For this review, take the finished solid that the model builds, in its own axes (mm). Face numbers are marked on the shaded views. A direction names the side the tool comes from. Coordinates: 2 decimals unless noted, no trailing zeros. Write each loop counter-clockwise with the first axis right and the second up, starting at its lowest first coordinate (ties: lowest second). Pieces come first, ordered by that corner, then holes. Notation, with made-up numbers: M 61.25,74 L 83.25,74 A31 cw 83.25,102 Z; hole C 15,-40 d8. An arc over 180 degrees is marked long. Return JSON: item names as keys, results as strings.
```python
from build123d import *

# Parameters (mm, degrees)
F0_W     = 99.4
F0_H     = 20
F1_DEPTH = 6
F2_W     = 5
F2_H     = 3.1
F2_W_2   = 6
F3_DEPTH = 6
F4_R     = 1.975
F5_DEPTH = 6
F6_W     = 30
F6_H     = 3
F7_DEPTH = 6


with BuildPart() as f1:
    # F0 (on Top) → F1 (new body)
    with BuildSketch(Plane.XY):
        Rectangle(F0_W, F0_H)
    extrude(amount=F1_DEPTH)

    # F2 (on face) → F3 (cut, through all)
    with BuildSketch(Plane.XY.offset(6)):
        with Locations((-47.2, 0)):
            Rectangle(F2_W, F2_H)
        with Locations((-41.7, 0)):
            Rectangle(F2_W_2, F2_H)
        with BuildLine():
            Line((-38.7, -1.55), (-44.7, -1.55))
            Line((-44.7, -1.55), (-44.7, -2.65))
            ThreePointArc((-44.7, -2.65), (-41.7, -5.65), (-38.7, -2.65))
            Line((-38.7, -2.65), (-38.7, -1.55))
        make_face()
        with BuildLine():
            Line((-44.7, 2.65), (-44.7, 1.55))
            Line((-44.7, 1.55), (-38.7, 1.55))
            Line((-38.7, 1.55), (-38.7, 2.65))
            ThreePointArc((-38.7, 2.65), (-41.7, 5.65), (-44.7, 2.65))
        make_face()
        with Locations((41.7, 0)):
            Rectangle(F2_W_2, F2_H)
        with BuildLine():
            Line((38.7, 2.65), (38.7, 1.55))
            Line((38.7, 1.55), (44.7, 1.55))
            Line((44.7, 1.55), (44.7, 2.65))
            ThreePointArc((44.7, 2.65), (41.7, 5.65), (38.7, 2.65))
        make_face()
        with BuildLine():
            Line((44.7, -1.55), (38.7, -1.55))
            Line((38.7, -1.55), (38.7, -2.65))
            ThreePointArc((38.7, -2.65), (41.7, -5.65), (44.7, -2.65))
            Line((44.7, -2.65), (44.7, -1.55))
        make_face()
        with Locations((47.2, 0)):
            Rectangle(F2_W, F2_H)
    extrude(amount=-F3_DEPTH, mode=Mode.SUBTRACT)

    # F4 (on face) → F5 (cut, through all)
    with BuildSketch(Plane.XY.offset(6)):
        Circle(F4_R)
    extrude(amount=-F5_DEPTH, mode=Mode.SUBTRACT)

    # F6 (on face) → F7 (cut, through all)
    with BuildSketch(Plane.XY.offset(6)):
        with Locations((-34.7, 8.5)):
            Rectangle(F6_W, F6_H)
    extrude(amount=-F7_DEPTH, mode=Mode.SUBTRACT)


solid = f1.part
```
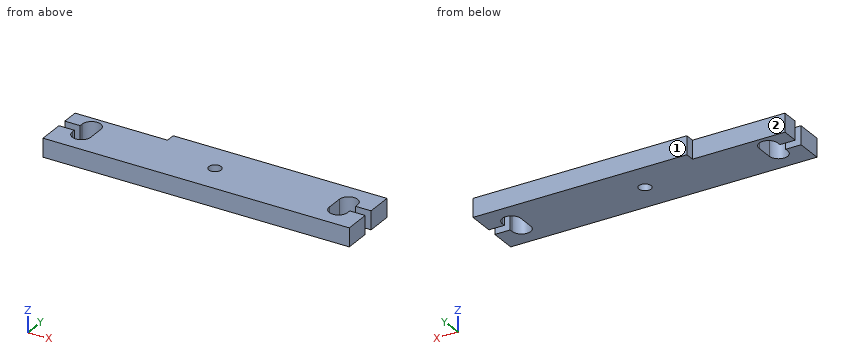
1. We need section A-A (x = 41.7). State the section outline as (y, z) points, plus the area to 3 significant figures.
Checks:
{"outline": "M -10,0 L -5.65,0 L -5.65,6 L -10,6 Z; M 5.65,0 L 10,0 L 10,6 L 5.65,6 Z", "area": "52.2 mm2"}
2. Clearance check with a flat-ended pin moving along its axis: pin 1 Ø1.5 at (x, z) = (-48, 3.5) entering from +Y. State where the tip first meets the part, or that it passes through.
Checks:
{"pin 1": "y = 7"}
3. We need section C-C (z = 1). State the section outline as (x, y) points (3 decimals), plus the area to 3 significant figures.
Checks:
{"outline": "M -49.7,-10 L 49.7,-10 L 49.7,-1.55 L 44.7,-1.55 L 44.7,-2.65 A3 cw 38.7,-2.65 L 38.7,2.65 A3 cw 44.7,2.65 L 44.7,1.55 L 49.7,1.55 L 49.7,10 L -19.7,10 L -19.7,7 L -49.7,7 L -49.7,1.55 L -44.7,1.55 L -44.7,2.65 A3 cw -38.7,2.65 L -38.7,-2.65 A3 cw -44.7,-2.65 L -44.7,-1.55 L -49.7,-1.55 Z; hole C 0,0 d3.95", "area": "1,730 mm2"}
4. Wall thickness on L1, parallel to X at y = -2.75, z = 1.9; L2, parallel to Y at x = 0, z = 1.55 (3 decimals); L3, parallel to X at y = 5.25, z = 1.55: over which ranges is each line inside the solid? List them lowest first. Write a range as from..to.
Checks:
{"L1": "-49.7..-44.7, -38.7..38.7, 44.7..49.7", "L2": "-10..-1.975, 1.975..10", "L3": "-49.7..-43.2, -40.2..40.2, 43.2..49.7"}
5. We need section B-B (y = 0). State the section outline as (x, z) points (3 decimals).
Checks:
{"outline": "M -38.7,0 L -1.975,0 L -1.975,6 L -38.7,6 Z; M 1.975,0 L 38.7,0 L 38.7,6 L 1.975,6 Z"}
6. For the marked faces 1 and 2, list the 3-axis set-ups (+Z, -Z, +X, -X, +Y, -Y) from which the entire face can be reached by the end or side of a thin tool; tool diameter is ignored.
Checks:
{"face 1": "+Z, -Z, +X, -X, +Y", "face 2": "+Z, -Z, -X, +Y"}
